For this review, take the finished solid that the model builds, in its own axes (mm). A direction names the side the tool comes from. Give positions to 0.01 mm unless a question says otherwise; leave off trailing zeros. Write each loop counter-clockwise with the first axis right and the second up, starting at its lowest first coordinate (ties: lowest second). Pieces come first, ordered by that corner, then holes.
1) We need section B-B on y = 6.5. Give the boundary of the cut face in (x, z).
2) We need section C-C on z = -6. Give the boundary of the cut face in (x, y), and give its area (3 significant figures).
3) Machinability: for faces 4 (the face through (6, -5.55, -22)), 5 (the face through (0, -13, 1)), 6 (the face through (11, 0, -10)), 7 (the face through (0.13, -15.59, -2.34)), which of the approach directions +Z, -Z, +X, -X, +Y, -Y give a long, thin tool a straight path to every point of the face, cutting with its end or side? Answer none if there is none.
4) Draft analysis for pull direction Y (two halves, no side actions). For faces 1 (the face through (0.6, 4, -22)), 2 (the face through (-12.399, 16.365, 0.937)), 3 (the face through (-9.85, 3, 3)), state which applies: pulls with the +Y half, pulls with the -Y half, needs draft (parallel to the pull), parting line crosses it, or undercut.
5) We need section A-A on z = -23. Give the boundary of the cut face in (x, y).
6) We need section D-D on y = -3. Give the boundary of the cut face in (x, z), and give its area (3 significant figures).
7) Wall thickness on line 1 along Y through (x, z) = (-5, -19.5); line 2 along Y through (x, z) = (-3.75, -8.5); line 3 along X through (y, z) = (7.5, -17.5): over which ranges is each line inside the solid? List them lowest first.
8) For P1, Ø3, axis at x = -6, z = -20, coming from the +Y side; P2, Ø2, axis at y = 12, z = -7, coming from the +X side; P3, Ø8, axis at x = 2, z = -20.5, coming from the -Y side, all flat-tipped, find the tip position at first contact; note any pin that passes through.
from build123d import *

# Parameters (mm, degrees)
SKETCH1_W           = 20
SKETCH1_H           = 26
EXTRUDE1_DEPTH      = 1.9
SKETCH2_W           = 22
SKETCH2_H           = 27.5
EXTRUDE2_DEPTH      = 17.2
SKETCH3_W           = 19.7
SKETCH3_H           = 25
EXTRUDE3_DEPTH      = 7.6
CUT_EXTRUDE1_DEPTH  = 19.7
SKETCH5_R           = 3
SKETCH5_R_2         = 2.2
SKETCH5_W           = 1.6
SKETCH5_H           = 5.5
CUT_EXTRUDE2_DEPTH  = 0.7
SKETCH6_R           = 80.623139619
CUT_EXTRUDE3_DEPTH  = 23.55
SKETCH7_W           = 6.35
SKETCH7_H           = 0.8
EXTRUDE4_DEPTH      = 10
CHAMFER1_SIZE       = 0.8
EXTRUDE5_DEPTH      = 9
EXTRUDE5_DEPTH_BACK = 9


with BuildPart() as part:
    # Sketch1 → Extrude1 (new body)
    with BuildSketch(Plane.XY):
        with BuildLine():
            Line((-11.7, -16.65), (11.7, -16.65))
            ThreePointArc((11.7, -16.65), (12.407106781, -16.357106781), (12.7, -15.65))
            Line((12.7, -15.65), (12.7, 15.65))
            ThreePointArc((12.7, 15.65), (12.407106781, 16.357106781), (11.7, 16.65))
            Line((11.7, 16.65), (-11.7, 16.65))
            ThreePointArc((-11.7, 16.65), (-12.407106781, 16.357106781), (-12.7, 15.65))
            Line((-12.7, 15.65), (-12.7, -15.65))
            ThreePointArc((-12.7, -15.65), (-12.407106781, -16.357106781), (-11.7, -16.65))
        make_face()
        Rectangle(SKETCH1_W, SKETCH1_H, mode=Mode.SUBTRACT)
    extrude(amount=EXTRUDE1_DEPTH)

    # Sketch2 → Extrude2 (add)
    with BuildSketch(Plane(origin=(0, 0, 0), x_dir=(-1, 0, 0), z_dir=(0, 0, -1))):
        Rectangle(SKETCH2_W, SKETCH2_H)
    extrude(amount=EXTRUDE2_DEPTH)

    # Sketch3 → Extrude3 (add)
    with BuildSketch(Plane.XY):
        Rectangle(SKETCH3_W, SKETCH3_H)
    extrude(amount=EXTRUDE3_DEPTH)

    # Sketch4 → Cut-Extrude1 (cut)
    with BuildSketch(Plane.ZY.offset(9.85)):
        with BuildLine():
            Line((0, -12.649110641), (10.2, -12.649110641))
            Line((10.2, -12.649110641), (10.2, 12.649110641))
            Line((10.2, 12.649110641), (0, 12.649110641))
            ThreePointArc((0, 12.649110641), (4.195359715, 10.827132519), (7.5, 7.664854858))
            Line((7.5, 7.664854858), (2.595963169, -11.733933535))
            ThreePointArc((2.595963169, -11.733933535), (1.322271739, -12.260422791), (0, -12.649110641))
        make_face()
    extrude(amount=-CUT_EXTRUDE1_DEPTH, mode=Mode.SUBTRACT)

    # Sketch5 → Cut-Extrude2 (cut)
    with BuildSketch(Plane(origin=(0, -1.321692682, 5.228190069), x_dir=(1, 0, 0), z_dir=(0, -0.245090789, 0.969500132))):
        with Locations((0, -7)):
            Circle(SKETCH5_R)
        with Locations((0, -7)):
            Circle(SKETCH5_R_2, mode=Mode.SUBTRACT)
        with Locations((0, 5.971443692)):
            Rectangle(SKETCH5_W, SKETCH5_H)
    extrude(amount=-CUT_EXTRUDE2_DEPTH, mode=Mode.SUBTRACT)

    # Sketch6 → Cut-Extrude3 (cut, through all)
    with BuildSketch(Plane.ZY.offset(9.85)):
        with Locations((82.607992112, -21.641802457)):
            Circle(SKETCH6_R)
    extrude(amount=-CUT_EXTRUDE3_DEPTH, mode=Mode.SUBTRACT)

    # Sketch7 → Extrude4 (add)
    with BuildSketch(Plane(origin=(0, 0, -17.2), x_dir=(-1, 0, 0), z_dir=(0, 0, -1))):
        Polygon((-0.6, -13.75), (0.6, -13.75), (0.6, -6.75), (11, -6.75), (11, -5.55), (0.6, -5.55), (0.6, 13.75), (-0.6, 13.75), (-0.6, -5.55), (-11, -5.55), (-11, -6.75), (-0.6, -6.75), align=None)
        with Locations((-5.475, 0.05)):
            Rectangle(SKETCH7_W, SKETCH7_H)
        with Locations((5.475, 0.05)):
            Rectangle(SKETCH7_W, SKETCH7_H)
        with Locations((-5.475, -11.65)):
            Rectangle(SKETCH7_W, SKETCH7_H)
        with Locations((5.475, -11.65)):
            Rectangle(SKETCH7_W, SKETCH7_H)
    extrude(amount=EXTRUDE4_DEPTH)

    # Chamfer1
    chamfer1_edges = [part.edges().sort_by_distance(p)[0] for p in [
        (8.65, 0.05, -27.2),
        (2.3, 0.05, -27.2),
        (-2.3, 0.05, -27.2),
        (-8.65, 0.05, -27.2),
        (8.65, -11.65, -27.2),
        (2.3, -11.65, -27.2),
        (-2.3, -11.65, -27.2),
        (-8.65, -11.65, -27.2),
    ]]
    chamfer(chamfer1_edges, length=CHAMFER1_SIZE)

    # Sketch8 → Extrude5 (add, two sides)
    with BuildSketch(Plane(origin=(0, 0, 0), x_dir=(0, 0, -1), z_dir=(1, 0, 0))) as extrude5_sk:
        Polygon((15.2, 13.75), (4.442640687, 16.95), (0.2, 16.25), (0.362790698, 15.263339375), (4.378231172, 15.925853253), (14.914876963, 12.791509075), align=None)
        Polygon((15.2, -13.75), (4.442640687, -16.95), (0.2, -16.25), (0.362790698, -15.263339375), (4.378231172, -15.925853253), (14.914876963, -12.791509075), align=None)
    extrude(amount=EXTRUDE5_DEPTH)
    extrude(extrude5_sk.sketch, amount=-EXTRUDE5_DEPTH_BACK)


solid = part.part
Results list:
1. outline: (-12.7, 0) - (-11, 0) - (-11, -17.2) - (-0.6, -17.2) - (-0.6, -27.2) - (0.6, -27.2) - (0.6, -17.2) - (11, -17.2) - (11, 0) - (12.7, 0) - (12.7, 1.9) - (10, 1.9) - (10, 0) - (9.85, 0) - (9.85, 7.06) - (0.8, 7.06) - (0.8, 6.48) - (-0.8, 6.48) - (-0.8, 7.06) - (-9.85, 7.06) - (-9.85, 0) - (-10, 0) - (-10, 1.9) - (-12.7, 1.9) - close
2. outline: (-11, -13.75) - (11, -13.75) - (11, 13.75) - (-11, 13.75) - close; (-9, -16.49) - (9, -16.49) - (9, -15.44) - (-9, -15.44) - close; (-9, 15.44) - (9, 15.44) - (9, 16.49) - (-9, 16.49) - close
2. area: 643 mm2
3. face 4: -Z, +X
3. face 5: +Z
3. face 6: -Z, +X, +Y, -Y
3. face 7: +X, -X
4. face 1: needs draft
4. face 2: pulls with the +Y half
4. face 3: undercut
5. outline: (-11, -6.75) - (-0.6, -6.75) - (-0.6, -13.75) - (0.6, -13.75) - (0.6, -6.75) - (11, -6.75) - (11, -5.55) - (0.6, -5.55) - (0.6, 13.75) - (-0.6, 13.75) - (-0.6, -5.55) - (-11, -5.55) - close; (-8.65, -12.05) - (-2.3, -12.05) - (-2.3, -11.25) - (-8.65, -11.25) - close; (-8.65, -0.35) - (-2.3, -0.35) - (-2.3, 0.45) - (-8.65, 0.45) - close; (2.3, -12.05) - (8.65, -12.05) - (8.65, -11.25) - (2.3, -11.25) - close; (2.3, -0.35) - (8.65, -0.35) - (8.65, 0.45) - (2.3, 0.45) - close
6. outline: (-12.7, 0) - (-11, 0) - (-11, -17.2) - (-0.6, -17.2) - (-0.6, -27.2) - (0.6, -27.2) - (0.6, -17.2) - (11, -17.2) - (11, 0) - (12.7, 0) - (12.7, 1.9) - (10, 1.9) - (10, 0) - (9.85, 0) - (9.85, 4.17) - (-9.85, 4.17) - (-9.85, 0) - (-10, 0) - (-10, 1.9) - (-12.7, 1.9) - close
6. area: 483 mm2
7. line 1: y = -12.05 to -11.25, -6.75 to -5.55, -0.35 to 0.45
7. line 2: y = -15.74 to -14.7, -13.75 to 13.75, 14.7 to 15.74
7. line 3: x = -0.6 to 0.6
8. P1: stops at y = 0.45
8. P2: stops at x = 11
8. P3: stops at y = -13.75
